Part model, mm, in its own coordinate system. A direction names the side the tool comes from. Coordinates: 2 decimals unless noted, no trailing zeros. Loops run counter-clockwise (first coordinate to the right, second up) from the corner with the lowest first, then second, coordinate; pieces in that order, holes last. Notation, with made-up numbers: (32, 59) - (69, 59) arc R10 ccw to (69, 77) - close; hole circle Ø9 at (83.25, 73). An arc over 180 degrees is marked (long way). Use a Markdown table: item, result. Add a question column.
1. Band-saw the part on D-D, the plane y = 13. Give the cut face in (x, z), plus the area to 3 significant figures.
2. Drop flat-ended pins along their axis: pin 1 (1 mm diameter, centred on x = 10.5, z = -16, fed in from -Y); pin 2 (1.5 mm diameter, centred on y = 29, z = 0.5, fed in from +X); pin 3 (9 mm diameter, centred on x = 8.5, z = 9, fed in from -Y). Give the stop position or say it passes through.
3. Wall check: probe 1 along Z at (x, y) = (7.5, 50.95); probe 2 along Y at (x, z) = (-3, -8); probe 3 along Y at (x, z) = (9.5, -15.5). Give the ranges that are in metal, low to high. Write a range as [from, to].
4. 3-axis set-ups, long thin cutter, end or side, ignore diameter. For faces 1 (the cylindrical face through (7.298, 2.028, 17.213)), 2 (the flat face through (10, 49.5, 0)), 3 (the cylindrical face through (-0.6, -9.93, -13.52)), 4 (the flat face through (6, 0, -20)): which of +Z, -Z, +X, -X, +Y, -Y reach the whole face in a straight line?
5. Band-saw the part on B-B, the plane x = 4.5. Give the cut face in (y, z).
6. Band-saw the part on A-A, the plane x = 7.5. Count the separate pieces of the cut face and the enclosed holes in it, plus the area to 3 significant figures.
7. Pull direction Z, two halves, no side cores. Call faces 5 (the cylindrical face through (-5.43, -9.9, 0.32)), 6 (the cylindrical face through (7.298, 51.472, 16.537)): pulls with the +Z half, pulls with the -Z half, needs draft (parallel to the pull), parting line crosses it, or undercut.
Autodesk Inventor part; units mm, degrees
ref_plane "YZ Plane" through (0, 0, 0) normal (1, 0, 0) x (0, 1, 0)
ref_plane "XZ Plane" through (0, 0, 0) normal (0, 1, 0) x (-1, 0, 0)
ref_plane "XY Plane" through (0, 0, 0) normal (0, 0, 1) x (1, 0, 0)
sketch "Sketch1" plane through (0, 0, 0) normal (0, 0, 1) x (1, 0, 0)
  line L0 (0, 0) -> (15, 0)
  line L1 (15, 0) -> (15, 4)
  line L2 (15, 4) -> (0, 4)
  line L3 (0, 4) -> (0, 0)
  line L4 (0, 53.5) -> (15, 53.5)
  line L5 (15, 53.5) -> (15, 49.5)
  line L6 (15, 49.5) -> (0, 49.5)
  line L7 (0, 49.5) -> (0, 53.5)
  line L8 (0, 53.5) -> (-6, 53.5)
  line L9 (-6, 53.5) -> (-6, -10.5)
  line L10 (-6, -10.5) -> (0, -10.5)
  line L11 (0, -10.5) -> (0, 53.5)
  point P0 (0, 49.5)
  dimension "d0" = 15
  dimension "d1" = 4
  dimension "d2" = 15
  dimension "d3" = 4
  dimension "d4" = 45.5
  dimension "d5" = 6
  dimension "d6" = 64
extrude "Extrusion1" add sketch "Sketch1" along normal mid plane 45
extrude "Extrusion2" cut sketch "Sketch1" along normal mid plane 30 contours L3 L2 L1 L0
sketch "Sketch3" plane through (0, 49.5, 22.5) normal (0, -1, 0) x (1, 0, 0)
  line L0 (0, 0) -> (15, 0)
  line L1 (7.5, 0) -> (7.5, -45)
  line L2 (15, -45) -> (0, -45)
  circle A0 centre (7.5, -3.75) radius 1.55
  circle A1 centre (7.5, -7.5) radius 1.55
  circle A2 centre (7.5, -22.5) radius 1.55
  circle A3 centre (7.5, -37.5) radius 1.55
  circle A4 centre (7.5, -41.25) radius 1.55
  line L3 (0, 0) -> (15, 0)
  line L4 (15, -45) -> (0, -45)
  line L5 (15, -45) -> (15, 0)
  point P0 (0, -22.5)
  dimension "d11" = 3.1
  dimension "d12" = 3.1
  dimension "d13" = 3.1
  dimension "d14" = 3.1
  dimension "d15" = 3.1
  dimension "d16" = 3.75
  dimension "d17" = 7.5
  dimension "d18" = 3.75
  dimension "d19" = 7.5
  dimension "d20" = 7.5
extrude "Extrusion3" cut sketch "Sketch3" along normal through all contours A0 L1 | L1 A0 | A4 L1 | L1 A4
extrude "Extrusion4" cut sketch "Sketch3" against normal through all contours A1 L1 | L1 A1 | A2 L1 | L1 A2 | A3 L1 | L1 A3
sketch "Sketch4" plane through (0, 4, -22.5) normal (1, 0, 0) x (0, 0, -1)
  circle A0 centre (-22.5, -1.5) radius 8 construction
  line L0 (-22.7792, 6.4951) -> (-22.2208, -9.4951) construction
  circle A1 centre (-22.7792, 6.4951) radius 1.55
  circle A2 centre (-22.5, -1.5) radius 4.5
  circle A3 centre (-22.5, -1.5) radius 12
  circle A4 centre (-29.5636, 2.2558) radius 1.55
  circle A5 centre (-29.2844, -5.7394) radius 1.55
  circle A6 centre (-22.2208, -9.4951) radius 1.55
  circle A7 centre (-15.4364, -5.2558) radius 1.55
  circle A8 centre (-15.7156, 2.7394) radius 1.55
  line L1 (-45, -14.5) -> (0, -14.5)
  line L2 (-22.5, -1.5) -> (-22.5, -14.5) construction
  point P0 (-22.5, -4)
  dimension "d25" = 16
  dimension "d26" = 3.1
  dimension "d29" = 9
  dimension "d30" = 24
  dimension "d33" = 360
  dimension "d43" = 13
  dimension "d44" = 2
extrude "Extrusion5" cut sketch "Sketch4" against normal blind 2.1
extrude "Extrusion6" cut sketch "Sketch4" against normal through all contours A1 | A2 | A4 | A5 | A6 | A7 | A8
fillet "Fillet1" radius 2 14 edges at (0, 49.5, 0) (15, 49.5, 0) (15, 53.5, 0) (-6, 53.5, 0) (0, 4, 18.75) (0, 4, -18.75) (15, 4, -18.75) (15, 0, -18.75) (15, 4, 18.75) (15, 0, 18.75) (0, -10.5, 0) (0, 0, 18.75) (0, 0, -18.75) (-6, -10.5, 0)
properties part number "MotorBracket" material "PC/ABS Plastic"
Geometry check:
| question | item | result |
|---|---|---|
| 1 | outline | (-6, -22.5) - (0, -22.5) - (0, -5.81) - (-2.1, -5.81) - (-2.1, 5.81) - (0, 5.81) - (0, 22.5) - (-6, 22.5) - close |
| 1 | area | 246 mm^2 |
| 2 | pin 1 | stops at y = 0 |
| 2 | pin 2 | stops at x = 0 |
| 2 | pin 3 | stops at y = 49.5 |
| 3 | probe 1 | z = [-22.5, -16.55], [-13.45, -1.55], [1.55, 13.45], [16.55, 22.5] |
| 3 | probe 2 | y = [-10.5, -2.49], [-0.02, 5.78], [7.7, 53.5] |
| 3 | probe 3 | y = [0, 4], [49.5, 53.5] |
| 4 | face 1 | -Y |
| 4 | face 2 | +Z, -Z, +X |
| 4 | face 3 | -Z, +X, -Y |
| 4 | face 4 | +Z, -Z, +X, -Y |
| 5 | outline | (0, -22.5) - (4, -22.5) - (4, -15) - (0, -15) - close; (0, 15) - (4, 15) - (4, 22.5) - (0, 22.5) - close; (49.5, -22.5) - (53.5, -22.5) - (53.5, 22.5) - (49.5, 22.5) - close |
| 6 | separate pieces | 8 |
| 6 | enclosed holes | 0 |
| 6 | area | 178 mm^2 |
| 7 | face 5 | needs draft |
| 7 | face 6 | undercut |
